Verification items for the finished model (mm, model axes). A direction names the side the tool comes from. Give positions to 0.01 mm unless a question says otherwise; leave off trailing zeros. Loops run counter-clockwise (first coordinate to the right, second up) from the corner with the lowest first, then second, coordinate; pieces in that order, holes last. Notation, with made-up numbers: M 42,67.5 L 46,67.5 A17 ccw 46,100.5 Z; hole C 47,1 d7. An arc over 180 degrees is marked long. Put each result on its own line as item: value. Start each with the question number.
from build123d import *

# Parameters (mm, degrees)
BOSS_EXTRU_1_DEPTH      = 4
ESQUISSE2_R             = 3.75
BOSS_EXTRU_3_DEPTH      = 1
BOSS_EXTRU_4_DEPTH      = 1
ENL_V_MAT_EXTRU_1_DEPTH = 82.630279309
CONG_1_R                = 1


with BuildPart() as part:
    # Esquisse1 → Boss.-Extru.1 (new body)
    with BuildSketch(Plane(origin=(0, 0, 0), x_dir=(1, 0, 0), z_dir=(0, 1, 0))):
        with BuildLine():
            Line((-65.8, 43.75), (65.8, 43.75))
            ThreePointArc((65.8, 43.75), (67.921320344, 42.871320344), (68.8, 40.75))
            Line((68.8, 40.75), (68.8, -40.75))
            ThreePointArc((68.8, -40.75), (67.921320344, -42.871320344), (65.8, -43.75))
            Line((65.8, -43.75), (-65.8, -43.75))
            ThreePointArc((-65.8, -43.75), (-67.921320344, -42.871320344), (-68.8, -40.75))
            Line((-68.8, -40.75), (-68.8, 40.75))
            ThreePointArc((-68.8, 40.75), (-67.921320344, 42.871320344), (-65.8, 43.75))
        make_face()
        with BuildLine():
            Line((-65.3, 42.75), (65.3, 42.75))
            ThreePointArc((65.3, 42.75), (67.067766953, 42.017766953), (67.8, 40.25))
            Line((67.8, 40.25), (67.8, -40.25))
            ThreePointArc((67.8, -40.25), (67.067766953, -42.017766953), (65.3, -42.75))
            Line((65.3, -42.75), (-65.3, -42.75))
            ThreePointArc((-65.3, -42.75), (-67.067766953, -42.017766953), (-67.8, -40.25))
            Line((-67.8, -40.25), (-67.8, 40.25))
            ThreePointArc((-67.8, 40.25), (-67.067766953, 42.017766953), (-65.3, 42.75))
        make_face(mode=Mode.SUBTRACT)
    extrude(amount=BOSS_EXTRU_1_DEPTH)

    # Esquisse2 → Boss.-Extru.3 (add)
    with BuildSketch(Plane(origin=(0, 4, 0), x_dir=(1, 0, 0), z_dir=(0, 1, 0))):
        with BuildLine():
            Line((31.185394692, 18.593528409), (67.917224545, 41.605916277))
            Line((67.917224545, 41.605916277), (67.067766953, 42.961800416))
            Line((67.067766953, 42.961800416), (30.320844752, 19.939957235))
            ThreePointArc((30.320844752, 19.939957235), (28.637181119, 21.166168316), (26.6, 21.6))
            Line((26.6, 21.6), (0.8, 21.6))
            Line((0.8, 21.6), (0.8, 43.322975794))
            Line((0.8, 43.322975794), (-0.8, 43.322975794))
            Line((-0.8, 43.322975794), (-0.8, 21.6))
            Line((-0.8, 21.6), (-26.6, 21.6))
            ThreePointArc((-26.6, 21.6), (-28.637181119, 21.166168316), (-30.320844752, 19.939957235))
            Line((-30.320844752, 19.939957235), (-67.067766953, 42.961800416))
            Line((-67.067766953, 42.961800416), (-67.917224545, 41.605916277))
            Line((-67.917224545, 41.605916277), (-31.185394692, 18.593528409))
            ThreePointArc((-31.185394692, 18.593528409), (-31.495251447, 17.618092958), (-31.6, 16.6))
            Line((-31.6, 16.6), (-31.6, 0.8))
            Line((-31.6, 0.8), (-68.322644777, 0.8))
            Line((-68.322644777, 0.8), (-68.322644777, -0.8))
            Line((-68.322644777, -0.8), (-31.6, -0.8))
            Line((-31.6, -0.8), (-31.6, -16.6))
            ThreePointArc((-31.6, -16.6), (-31.495251447, -17.618092958), (-31.185394692, -18.593528409))
            Line((-31.185394692, -18.593528409), (-67.921921264, -41.608858758))
            Line((-67.921921264, -41.608858758), (-67.072463672, -42.964742898))
            Line((-67.072463672, -42.964742898), (-30.320844752, -19.939957235))
            ThreePointArc((-30.320844752, -19.939957235), (-28.637181119, -21.166168316), (-26.6, -21.6))
            Line((-26.6, -21.6), (-0.8, -21.6))
            Line((-0.8, -21.6), (-0.8, -43.218261979))
            Line((-0.8, -43.218261979), (0.8, -43.218261979))
            Line((0.8, -43.218261979), (0.8, -21.6))
            Line((0.8, -21.6), (26.6, -21.6))
            ThreePointArc((26.6, -21.6), (28.637181119, -21.166168316), (30.320844752, -19.939957235))
            Line((30.320844752, -19.939957235), (66.872148546, -42.839246036))
            Line((66.872148546, -42.839246036), (67.721606138, -41.483361896))
            Line((67.721606138, -41.483361896), (31.185394692, -18.593528409))
            ThreePointArc((31.185394692, -18.593528409), (31.495251447, -17.618092958), (31.6, -16.6))
            Line((31.6, -16.6), (31.6, -0.8))
            Line((31.6, -0.8), (68.284636361, -0.8))
            Line((68.284636361, -0.8), (68.284636361, 0.8))
            Line((68.284636361, 0.8), (31.6, 0.8))
            Line((31.6, 0.8), (31.6, 16.6))
            ThreePointArc((31.6, 16.6), (31.495251447, 17.618092958), (31.185394692, 18.593528409))
        make_face()
        with Locations(Location((0, 0, 0), (0, 0, 270))):
            Circle(ESQUISSE2_R, mode=Mode.SUBTRACT)
        with BuildLine():
            Line((-26, 20), (-0.8, 20))
            Line((-0.8, 20), (-0.8, 5.289848769))
            ThreePointArc((-0.8, 5.289848769), (-5.35, 0), (-0.8, -5.289848769))
            Line((-0.8, -5.289848769), (-0.8, -20))
            Line((-0.8, -20), (-26, -20))
            ThreePointArc((-26, -20), (-28.828427125, -18.828427125), (-30, -16))
            Line((-30, -16), (-30, 16))
            ThreePointArc((-30, 16), (-28.828427125, 18.828427125), (-26, 20))
        make_face(mode=Mode.SUBTRACT)
        with BuildLine():
            Line((30, 16), (30, -16))
            ThreePointArc((30, -16), (29.91194143, -16.834694103), (29.651642878, -17.632637221))
            Line((29.651642878, -17.632637221), (4.907492575, -2.130496802))
            ThreePointArc((4.907492575, -2.130496802), (5.35, 0), (4.907492575, 2.130496802))
            Line((4.907492575, 2.130496802), (29.651642878, 17.632637221))
            ThreePointArc((29.651642878, 17.632637221), (29.91194143, 16.834694103), (30, 16))
        make_face(mode=Mode.SUBTRACT)
        with BuildLine():
            Line((0.8, 20), (0.8, 5.289848769))
            ThreePointArc((0.8, 5.289848769), (2.590994023, 4.680731778), (4.058034983, 3.486380942))
            Line((4.058034983, 3.486380942), (28.717305938, 18.935344688))
            ThreePointArc((28.717305938, 18.935344688), (27.459215756, 19.724337441), (26, 20))
            Line((26, 20), (0.8, 20))
        make_face(mode=Mode.SUBTRACT)
        with BuildLine():
            Line((0.8, -20), (0.8, -5.289848769))
            ThreePointArc((0.8, -5.289848769), (2.590994023, -4.680731778), (4.058034983, -3.486380942))
            Line((4.058034983, -3.486380942), (28.717305938, -18.935344688))
            ThreePointArc((28.717305938, -18.935344688), (27.459215756, -19.724337441), (26, -20))
            Line((26, -20), (0.8, -20))
        make_face(mode=Mode.SUBTRACT)
    extrude(amount=-BOSS_EXTRU_3_DEPTH)

    # Esquisse3 → Boss.-Extru.4 (add)
    with BuildSketch(Plane(origin=(0, 4, 0), x_dir=(1, 0, 0), z_dir=(0, 1, 0))):
        with BuildLine():
            Line((-31.6, 7.246102482), (-30, 7.246102482))
            Line((-30, 7.246102482), (-30, -10.710151561))
            Line((-30, -10.710151561), (-31.6, -10.710151561))
            Line((-31.6, -10.710151561), (-31.6, -3.4))
            Line((-31.6, -3.4), (-36.8, -3.4))
            ThreePointArc((-36.8, -3.4), (-40.2, 0), (-36.8, 3.4))
            Line((-36.8, 3.4), (-31.6, 3.4))
            Line((-31.6, 3.4), (-31.6, 7.246102482))
        make_face()
        with BuildLine():
            Line((-36.8, 1.8), (-33.91555898, 1.8))
            Line((-33.91555898, 1.8), (-31.6, 1.8))
            Line((-31.6, 1.8), (-31.6, -1.8))
            Line((-31.6, -1.8), (-33.91555898, -1.8))
            Line((-33.91555898, -1.8), (-36.8, -1.8))
            ThreePointArc((-36.8, -1.8), (-38.6, 0), (-36.8, 1.8))
        make_face(mode=Mode.SUBTRACT)
    extrude(amount=-BOSS_EXTRU_4_DEPTH)

    # Esquisse4 → Enlèv. mat.-Extru.1 (cut, through all)
    with BuildSketch(Plane(origin=(0, 4, 0), x_dir=(1, 0, 0), z_dir=(0, 1, 0))):
        with BuildLine():
            Line((-36.8, 1.8), (-28.230544018, 1.8))
            Line((-28.230544018, 1.8), (-28.230544018, -1.8))
            Line((-28.230544018, -1.8), (-36.8, -1.8))
            ThreePointArc((-36.8, -1.8), (-38.6, 0), (-36.8, 1.8))
        make_face()
    extrude(amount=-ENL_V_MAT_EXTRU_1_DEPTH, mode=Mode.SUBTRACT)

    # Congé1
    cong_1_edges = [part.edges().sort_by_distance(p)[0] for p in [
        (-30, 3.5, -1.8),
        (-30, 3.5, 1.8),
    ]]
    fillet(cong_1_edges, radius=CONG_1_R)


solid = part.part
Q1. Cross-section at B-B, the plane x = 35. Record the boundary of the cut face in (y, z), then the cut area to 3 significant figures.
Q2. Set-up check for faces 5 (the face through (-48.09, 3.51, -31.07)), 6 (the face through (5, 4, 0)): record each of +Z, -Z, +X, -X, +Y, -Y from which the full face is reachable in a straight line by a thin tool's end or side.
Q3. Cross-section at A-A, the plane y = 1.8. Record the boundary of the cut face in (x, z), then the cut area to 3 significant figures.
Q4. Release check for a two-part mould opening along X. For faces 1 (the face through (-68.8, 2, 1)), 2 (the face through (1, 2, 43.75)), 3 (the face through (-38.88, 3.51, 2.69)), 4 (the face through (-5.35, 3.51, -0.11)) record: pulls with the +X half, pulls with the -X half, needs draft (parallel to the pull), parting line crosses it, or undercut.
Q5. Cross-section at C-C, the plane z = 10.5. Record the boundary of the cut face in (x, y), then the cut area to 3 significant figures.
Q6. Go/stop test with flat-tipped pins: pin 1 (10 mm diameter, centred on x = -49.5, z = 24.5, fed in from -Y); pin 2 (6 mm diameter, centred on x = 0, z = 0, fed in from -Y). Record where each tip stops, or that it passes through.
Q7. Scan lines: L1, parallel to X at y = 1.25, z = 30; L2, parallel to Z at x = 59, y = 1.4; L3, parallel to Z at x = -43, y = 3.45. Record each from-to range of solid material in increasing order.
Q8. Cross-section at D-D, the plane x = 8.5. Record the boundary of the cut face in (y, z).
Ans:
1. outline: M 0,-43.75 L 4,-43.75 L 4,-42.75 L 0,-42.75 Z; M 0,42.75 L 4,42.75 L 4,43.75 L 0,43.75 Z; M 3,-22.87 L 4,-22.87 L 4,-20.98 L 3,-20.98 Z; M 3,-0.8 L 4,-0.8 L 4,0.8 L 3,0.8 Z; M 3,20.98 L 4,20.98 L 4,22.87 L 3,22.87 Z
1. area: 13.4 mm^2
2. face 5: +Y, -Y
2. face 6: +Z, -Z, +X, -X, +Y
3. outline: M -68.8,-40.75 A3 ccw -65.8,-43.75 L 65.8,-43.75 A3 ccw 68.8,-40.75 L 68.8,40.75 A3 ccw 65.8,43.75 L -65.8,43.75 A3 ccw -68.8,40.75 Z; hole M -67.8,-40.25 A2.5 ccw -65.3,-42.75 L 65.3,-42.75 A2.5 ccw 67.8,-40.25 L 67.8,40.25 A2.5 ccw 65.3,42.75 L -65.3,42.75 A2.5 ccw -67.8,40.25 Z
3. area: 444 mm^2
4. face 1: pulls with the -X half
4. face 2: needs draft
4. face 3: undercut
4. face 4: undercut
5. outline: M -68.8,0 L -67.8,0 L -67.8,4 L -68.8,4 Z; M -31.6,3 L -30,3 L -30,4 L -31.6,4 Z; M -0.8,3 L 0.8,3 L 0.8,4 L -0.8,4 Z; M 15.25,3 L 18.27,3 L 18.27,4 L 15.25,4 Z; M 30,3 L 31.6,3 L 31.6,4 L 30,4 Z; M 67.8,0 L 68.8,0 L 68.8,4 L 67.8,4 Z
5. area: 15.8 mm^2
6. pin 1: stops at y = 3
6. pin 2: passes through
7. L1: x = -68.8 to -67.8, 67.8 to 68.8
7. L2: z = -43.75 to -42.75, 42.75 to 43.75
7. L3: z = -43.75 to -42.75, -27.88 to -26, -0.8 to 0.8, 26 to 27.88, 42.75 to 43.75
8. outline: M 0,-43.75 L 4,-43.75 L 4,-42.75 L 0,-42.75 Z; M 0,42.75 L 4,42.75 L 4,43.75 L 0,43.75 Z; M 3,-21.6 L 4,-21.6 L 4,-20 L 3,-20 Z; M 3,-6.27 L 4,-6.27 L 4,-4.38 L 3,-4.38 Z; M 3,4.38 L 4,4.38 L 4,6.27 L 3,6.27 Z; M 3,20 L 4,20 L 4,21.6 L 3,21.6 Z
